from build123d import *

# Parameters (mm, degrees)
F0_W     = 20
F0_H     = 25
F1_DEPTH = 80
F2_R     = 5
F2_R_2   = 4.5
F3_DEPTH = 25
F4_W     = 20
F4_H     = 20
F5_DEPTH = 70
F6_W     = 20
F6_H     = 45
F7_DEPTH = 15
F8_R     = 5
F9_DEPTH = 30
F10_SIZE = 2


with BuildPart() as f1:
    # F0 (on Top) → F1 (new body)
    with BuildSketch(Plane.XY):
        with Locations((10, -12.5)):
            Rectangle(F0_W, F0_H)
    extrude(amount=F1_DEPTH)

    # F2 (on face) → F3 (cut)
    with BuildSketch(Plane.YZ.offset(20)):
        with Locations((-12.5, 71)):
            Circle(F2_R)
        with Locations((-12.5, 56)):
            Circle(F2_R_2)
        with Locations((-12.5, 41)):
            Circle(F2_R)
        with Locations((-12.5, 26)):
            Circle(F2_R_2)
    extrude(amount=-F3_DEPTH, mode=Mode.SUBTRACT)

    # F4 (on face) → F5 (join)
    with BuildSketch(Plane(origin=(0, 0, 0), x_dir=(-1, 0, 0), z_dir=(0, 1, 0))):
        with Locations((-10, 10)):
            Rectangle(F4_W, F4_H)
    extrude(amount=F5_DEPTH)

    # F6 (on face) → F7 (join)
    with BuildSketch(Plane(origin=(0, 70, 0), x_dir=(-1, 0, 0), z_dir=(0, 1, 0))):
        with Locations((-10, -2.5)):
            Rectangle(F6_W, F6_H)
    extrude(amount=F7_DEPTH)

    # F8 (on face) → F9 (join)
    with BuildSketch(Plane(origin=(0, 85, 0), x_dir=(-1, 0, 0), z_dir=(0, 1, 0))):
        with Locations((-10, -15)):
            Circle(F8_R)
    extrude(amount=F9_DEPTH)

    # F10
    f10_edges = [f1.edges().sort_by_distance(p)[0] for p in [
        (15, 115, -15),
    ]]
    chamfer(f10_edges, length=F10_SIZE)


solid = f1.part
Model file for the job. Use its own axes, mm. A direction names the side the tool comes from. Give positions to 0.01 mm unless a question says otherwise; leave off trailing zeros. Loops run counter-clockwise (first coordinate to the right, second up) from the corner with the lowest first, then second, coordinate; pieces in that order, holes last.
1) Saw through at B-B (y = -12.5). Write the cut outline in (x, z).
2) Wall check: line 1 (Z direction, x = 11.5, y = -12.5); line 2 (Y direction, x = 1, z = 26.5); line 3 (Z direction, x = 17.25, y = 81). Give the ranges that are in metal, low to high.
3) Saw through at D-D (z = 56). Write the cut outline in (x, y), plus the area to 3 significant figures.
4) Pull direction Y, two halves, no side cores. Call faces 6 (the flat face through (10, 22, 0)), 7 (the flat face through (10, -25, 39)), 8 (the cylindrical face through (10.14, -9.812, 45.216)): +Y half, -Y half, draft (parallel to the pull), parting line (faces both ways), or undercut.
5) Saw through at A-A (z = 41). Write the cut outline in (x, y), plus the area to 3 significant figures.
6) Tool access for faces 1 (the cylindrical face through (10.14, -10.081, 29.794)), 2 (the cylindrical face through (7.693, 98.804, -19.436)), 3 (the flat face through (10, 77, -25)), 4 (the flat face through (10, 0, 50)), 5 (the flat face through (10, 70, -12)): list every direction of +Z, -Z, +X, -X, +Y, -Y with a clear straight run to the whole face (end or side of a thin tool).
7) Saw through at C-C (x = 18). Write the cut outline in (y, z).
8) Flat gauge pins, fed straight in: pin 1 Ø6 at (x, z) = (5, 11) entering from +Y; pin 2 Ø6 at (x, y) = (12, 42) entering from +Z; pin 3 Ø10 at (x, z) = (8, 45.5) entering from +Y. Where does each tip first touch, or does it go through?
Answer block:
1. outline: (0, 0) - (20, 0) - (20, 21.5) - (0, 21.5) - close; (0, 30.5) - (20, 30.5) - (20, 36) - (0, 36) - close; (0, 46) - (20, 46) - (20, 51.5) - (0, 51.5) - close; (0, 60.5) - (20, 60.5) - (20, 66) - (0, 66) - close; (0, 76) - (20, 76) - (20, 80) - (0, 80) - close
2. line 1: z = 0 to 21.5, 30.5 to 36, 46 to 51.5, 60.5 to 66, 76 to 80
2. line 2: y = -25 to -16.97, -8.03 to 0
2. line 3: z = -25 to 20
3. outline: (0, -25) - (20, -25) - (20, -17) - (0, -17) - close; (0, -8) - (20, -8) - (20, 0) - (0, 0) - close
3. area: 320 mm2
4. face 6: draft
4. face 7: -Y half
4. face 8: undercut
5. outline: (0, -25) - (20, -25) - (20, -17.5) - (0, -17.5) - close; (0, -7.5) - (20, -7.5) - (20, 0) - (0, 0) - close
5. area: 300 mm2
6. face 1: +X, -X
6. face 2: +Y
6. face 3: -Z, +X, -X, +Y, -Y
6. face 4: +Z, +X, -X, +Y
6. face 5: -Z, +X, -X, -Y
7. outline: (-25, 0) - (70, 0) - (70, -25) - (85, -25) - (85, 20) - (0, 20) - (0, 80) - (-25, 80) - close; hole circle Ø10 at (-12.5, 41); hole circle Ø10 at (-12.5, 71); hole circle Ø9 at (-12.5, 26); hole circle Ø9 at (-12.5, 56)
8. pin 1: stops at y = 85
8. pin 2: stops at z = 20
8. pin 3: stops at y = 0
